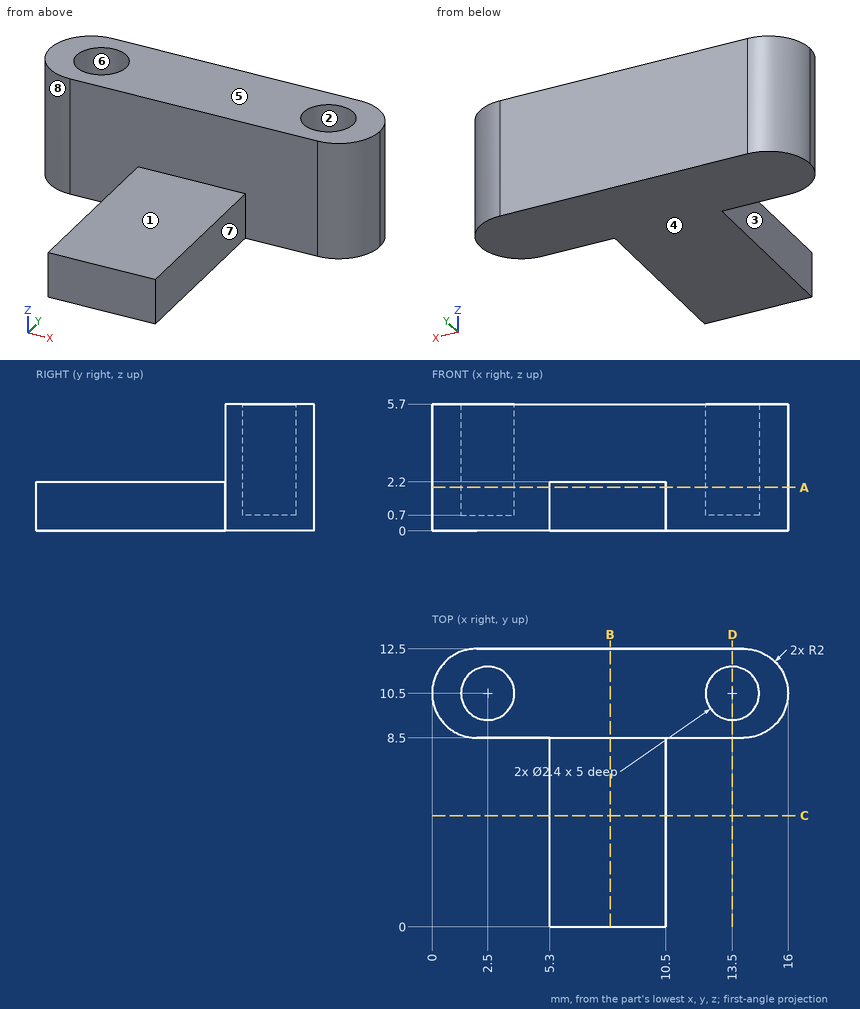
Input: dimensioned drawing with shaded views. Units: mm. Origin: part minimum x, y, z. A direction names the side the tool comes from. Coordinates: 2 decimals unless noted, no trailing zeros. Write each loop counter-clockwise with the first axis right and the second up, starting at its lowest first coordinate (ties: lowest second). Pieces come first, ordered by that corner, then holes. Notation, with made-up numbers: (87.25, 0.5) -> (118.25, 0.5) arc R24 cw to (118.25, 32.5) -> close; hole circle Ø4 at (29.5, -23.75). An arc over 180 degrees is marked (long way). Return JSON: item names as keys, results as strings. Group by question number.
1) Set-up query: the marked faces 1, 2, 3 and 4. Return all of +Z, -Z, +X, -X, +Y, -Y with unobstructed straight access to the full face (end or side cutting, diameter ignored); none if empty.
2) Ray query, line 1 along Y through (x, z) = (13.5, 2.25); line 2 along Y through (x, z) = (11.75, 3.45); line 3 along X through (y, z) = (11.5, 3). Return the intervals inside material, ascending.
3) Contact query for flat-ended pins moving along their axis: P1, Ø3, axis at x = 13.5, y = 10.5, coming from the -Z side; P2, Ø0.7, axis at x = 13.5, y = 10, coming from the +Z side; P3, Ø1.6, axis at x = 9, y = 4.5, coming from the +Z side; P4, Ø0.7, axis at y = 3.5, z = 1, coming from the +X side. Output: stop coordinate, or through.
4) Section query A-A, the plane z = 1.95. State how many separate pieces and enclosed holes the cut face has, plus the area to 3 significant figures.
5) Section query C-C, the plane y = 5. Return loops of the section in (x, z), plus the area to 3 significant figures.
6) Section query B-B, the plane x = 8. Return loops of the section in (y, z), plus the area to 3 significant figures.
7) Section query D-D, the plane x = 13.5. Return loops of the section in (y, z).
8) Mould query, pull axis X, two halves, no side actions, for the marked faces 5, 6, 7 and 8. Classes: +X half, -X half, draft (parallel to the pull), parting line (faces both ways), or undercut.
From the geometry:
{
 "1": {"face 1": "+Z, +X, -X, -Y", "face 2": "+Z", "face 3": "+Z, -Z, -X, -Y", "face 4": "-Z, +X, -X, +Y, -Y"},
 "2": {"line 1": "8.5 to 9.3, 11.7 to 12.5", "line 2": "8.5 to 12.5", "line 3": "0.27 to 1.84, 3.16 to 12.84, 14.16 to 15.73"},
 "3": {"P1": "z = 0", "P2": "z = 0.7", "P3": "z = 2.2", "P4": "x = 10.5"},
 "4": {"separate pieces": "1", "enclosed holes": "2", "area": "95.7 mm²"},
 "5": {"outline": "(5.3, 0) -> (10.5, 0) -> (10.5, 2.2) -> (5.3, 2.2) -> close", "area": "11.4 mm²"},
 "6": {"outline": "(0, 0) -> (12.5, 0) -> (12.5, 5.7) -> (8.5, 5.7) -> (8.5, 2.2) -> (0, 2.2) -> close", "area": "41.5 mm²"},
 "7": {"outline": "(8.5, 0) -> (12.5, 0) -> (12.5, 5.7) -> (11.7, 5.7) -> (11.7, 0.7) -> (9.3, 0.7) -> (9.3, 5.7) -> (8.5, 5.7) -> close"},
 "8": {"face 5": "draft", "face 6": "undercut", "face 7": "+X half", "face 8": "-X half"}
}
